Can you work these out from the model? Positions are in its coordinate system, mm. Face numbers are marked on the shaded views. A direction names the side the tool comes from. Give positions to 0.01 mm unless a question says otherwise; leave off trailing zeros. Order: outer loops, then holes, each group sorted by start corner. A loop starts at its lowest first (then second) coordinate and runs counter-clockwise, first axis right, second up. Notation, with made-up numbers: (62, -1) - (86, -1) arc R16 ccw to (86, 17) - close; hole circle Ø9 at (-26, 12.5). An arc over 180 degrees is marked (long way). Return JSON: item names as keys, results as strings.
```python
from build123d import *

# Parameters (mm, degrees)
SKETCH2_OUTSIDE_W  = 54.332
SKETCH2_OUTSIDE_H  = 54.332
CUT_EXTRUDE2_DEPTH = 69.393971984


with BuildPart() as part:
    # Sketch1 → Revolve2 (revolve)
    with BuildSketch(Plane.XY, mode=Mode.PRIVATE) as revolve2_sk:
        Polygon((0, 0), (6.749601751, 2.795776586), (13.028153792, 7.138607178), (18.025292424, 12.467968867), (18.025292424, 37.870552131), (10.605112725, 41.454777816), (2.54, 43.145841757), (2.54, 63.465841757), (0, 63.465841757), align=None)
    revolve(revolve2_sk.sketch.rotate(Axis((0, 63.465841757, 0), (0, -1, 0)), 90), axis=Axis((0, 63.465841757, 0), (0, -1, 0)))

    # Sketch2 outside → Cut-Extrude2 (cut, through all)
    with BuildSketch(Plane(origin=(0, 63.465841757, 0), x_dir=(1, 0, 0), z_dir=(0, 1, 0))):
        Rectangle(SKETCH2_OUTSIDE_W, SKETCH2_OUTSIDE_H)
        Polygon((-10.595001055, 14.582767899), (-14.582767899, 10.595001055), (-17.143071818, 5.570121687), (-18.025292424, 0), (-17.143071818, -5.570121687), (-14.582767899, -10.595001055), (-10.595001055, -14.582767899), (-5.570121687, -17.143071818), (0, -18.025292424), (5.570121687, -17.143071818), (10.595001055, -14.582767899), (14.582767899, -10.595001055), (17.143071818, -5.570121687), (18.025292424, 0), (17.143071818, 5.570121687), (14.582767899, 10.595001055), (10.595001055, 14.582767899), (5.570121687, 17.143071818), (0, 18.025292424), (-5.570121687, 17.143071818), align=None, mode=Mode.SUBTRACT)
    extrude(amount=-CUT_EXTRUDE2_DEPTH, mode=Mode.SUBTRACT)


solid = part.part
```
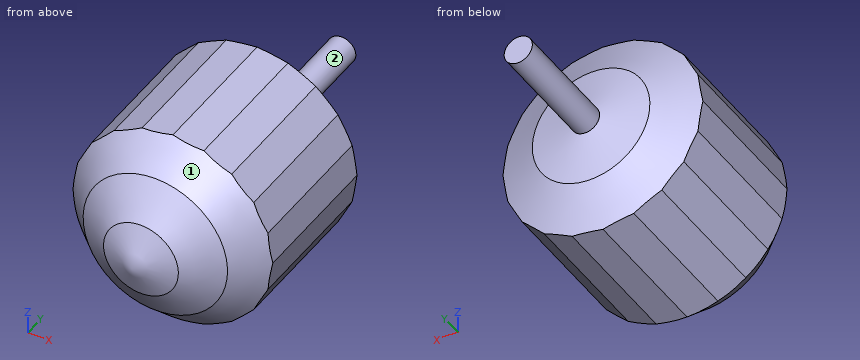
1. On a 3-axis mill with a long thin cutter (end or side, diameter ignored), from which of +Z, -Z, +X, -X, +Y, -Y can I reach the whole of each face in a straight line? I mean the marked faces 1 and 2. Say none if no direction works.
Checks:
{"face 1": "-Y", "face 2": "+Y"}
2. Suppose I cut it at A-A (y = 21). List the corners of the cut face in (x, z) for me (3 decimals), plus the area to 3 significant figures.
Checks:
{"outline": "(-18.025, 0) - (-17.143, -5.57) - (-14.583, -10.595) - (-10.595, -14.583) - (-5.57, -17.143) - (0, -18.025) - (5.57, -17.143) - (10.595, -14.583) - (14.583, -10.595) - (17.143, -5.57) - (18.025, 0) - (17.143, 5.57) - (14.583, 10.595) - (10.595, 14.583) - (5.57, 17.143) - (0, 18.025) - (-5.57, 17.143) - (-10.595, 14.583) - (-14.583, 10.595) - (-17.143, 5.57) - close", "area": "1,000 mm^2"}
3. For pin 1 Ø5 at (x, y) = (10.5, 19) entering from -Z (3 decimals); pin 2 Ø5 at (y, z) = (6.5, 7) entering from -X; pin 3 Ø6 at (y, z) = (49.5, 2.5) entering from +X, each with a flat end and sliding along its axis, tell me the tip position at first contact or that it passes through.
Checks:
{"pin 1": "z = -15.905", "pin 2": "x = -13.29", "pin 3": "x = 2.54"}
4. If I drill on L1, parallel to Z at x = -7, y = 10.5; L2, parallel to Z at x = -3.5, y = 6; L3, parallel to X at y = 39, z = -1, over which ranges is the centre line in solid material (lowest first)? Write a range as [from, to].
Checks:
{"L1": "[-14.59, 14.59]", "L2": "[-10.83, 10.83]", "L3": "[-15.66, 15.66]"}
